Verification items for the finished model (mm, model axes). A direction names the side the tool comes from. Give positions to 0.01 mm unless a question says otherwise; leave off trailing zeros. Order: outer loops, then holes, each group sorted by start corner. A loop starts at its lowest first (then second) coordinate and runs counter-clockwise, first axis right, second up. Notation, with made-up numbers: M 43.5,-5 L 76.5,-5 A11 cw 76.5,-1 Z; hole C -32.75,26.5 d4. An arc over 180 degrees is marked long. Answer as a JSON object with one key per item and string values.
```python
from build123d import *

# Parameters (mm, degrees)
SKETCH_1_R          = 1
EXTRUDE_1_DEPTH     = 3.3
SKETCH_2_W          = 20
SKETCH_2_H          = 8
CUT_EXTRUDE_1_DEPTH = 2.2
FILLET_1_R          = 1
EXTRUDE_2_DEPTH     = 2


with BuildPart() as part:
    # 草图1 → 凸台-拉伸1 (new body)
    with BuildSketch(Plane.XY):
        with BuildLine():
            Line((10.5, -13.638181697), (10.5, -22.5))
            ThreePointArc((10.5, -22.5), (0, -33), (-10.5, -22.5))
            Line((-10.5, -22.5), (-10.5, -13.638181697))
            ThreePointArc((-10.5, -13.638181697), (-7.5, 0), (-10.5, 13.638181697))
            Line((-10.5, 13.638181697), (-10.5, 22.5))
            ThreePointArc((-10.5, 22.5), (0, 33), (10.5, 22.5))
            Line((10.5, 22.5), (10.5, 13.638181697))
            ThreePointArc((10.5, 13.638181697), (7.5, 0), (10.5, -13.638181697))
        make_face()
        with Locations((0, 7)):
            Circle(SKETCH_1_R, mode=Mode.SUBTRACT)
        with Locations((0, -7)):
            Circle(SKETCH_1_R, mode=Mode.SUBTRACT)
        with Locations((-6, 28.25)):
            Circle(SKETCH_1_R, mode=Mode.SUBTRACT)
        with Locations((6, 28.25)):
            Circle(SKETCH_1_R, mode=Mode.SUBTRACT)
        with Locations((6, -28.25)):
            Circle(SKETCH_1_R, mode=Mode.SUBTRACT)
        with Locations((-6, -28.25)):
            Circle(SKETCH_1_R, mode=Mode.SUBTRACT)
        with BuildLine():
            Line((-4, -22.499999544), (-4, -8.5))
            Line((-4, -8.5), (4, -8.5))
            Line((4, -8.5), (4, -22.500000456))
            ThreePointArc((4, -22.500000456), (-4.56e-07, -26.5), (-4, -22.499999544))
        make_face(mode=Mode.SUBTRACT)
        with BuildLine():
            Line((-4, 22.499999544), (-4, 8.5))
            Line((-4, 8.5), (4, 8.5))
            Line((4, 8.5), (4, 22.500000456))
            ThreePointArc((4, 22.500000456), (-4.56e-07, 26.5), (-4, 22.499999544))
        make_face(mode=Mode.SUBTRACT)
    extrude(amount=EXTRUDE_1_DEPTH)

    # 草图2 → 切除-拉伸1 (cut)
    with BuildSketch(Plane.XY.offset(3.3)):
        Polygon((-3.8, 24.3), (-2.871447866, 34.3), (2.871447866, 34.3), (3.8, 24.3), (8.25, 24.3), (8.25, 17.8), (-8.25, 17.8), (-8.25, 24.3), align=None)
        Rectangle(SKETCH_2_W, SKETCH_2_H)
        Polygon((3.8, -24.3), (8.25, -24.3), (8.25, -17.8), (-8.25, -17.8), (-8.25, -24.3), (-3.8, -24.3), (-2.871447866, -34.3), (2.871447866, -34.3), align=None)
    extrude(amount=-CUT_EXTRUDE_1_DEPTH, mode=Mode.SUBTRACT)

    # 圆角1
    fillet_1_edges = [part.edges().sort_by_distance(p)[0] for p in [
        (0, -4, 1.1),
        (0, 4, 1.1),
        (0, -4, 3.3),
        (0, 4, 3.3),
    ]]
    fillet(fillet_1_edges, radius=FILLET_1_R)

    # 草图3 → 凸台-拉伸2 (add)
    with BuildSketch(Plane(origin=(0, 8.5, 0), x_dir=(1, 0, 0), z_dir=(0, 1, 0))):
        with BuildLine():
            Line((-3, -3.3), (3, -3.3))
            ThreePointArc((3, -3.3), (0, -0.3), (-3, -3.3))
        make_face()
    extrude_2 = extrude(amount=EXTRUDE_2_DEPTH)

    # 镜向1: 凸台-拉伸2 across plane
    add(extrude_2.mirror(Plane.ZX))


solid = part.part
```
Q1. Section check D-D on y = -28.25. Record the cut outline in (x, z), then the cut area to 3 significant figures.
Resolved:
{"outline": "M -8.79,0 L -7,0 L -7,3.3 L -8.79,3.3 Z; M -5,0 L 5,0 L 5,3.3 L 3.43,3.3 L 3.43,1.1 L -3.43,1.1 L -3.43,3.3 L -5,3.3 Z; M 7,0 L 8.79,0 L 8.79,3.3 L 7,3.3 Z", "area": "29.7 mm²"}
Q2. Gauge pin test, flat ends, axial feed: pin 1 Ø5 at (x, y) = (2.5, -0.5) entering from +Z; pin 2 Ø1 at (y, z) = (6.5, 1) entering from +X; pin 3 Ø1.1 at (x, z) = (-6, 1.5) entering from +Y. Record the tip position at first contact, or that the pin passes through.
Resolved:
{"pin 1": "stops at z = 1.1", "pin 2": "stops at x = 8.26", "pin 3": "stops at y = 31.47"}
Q3. Material ranges on L1, parallel to Y at x = 0, z = 0.95; L2, parallel to Y at x = 6, z = 1.8; L3, parallel to X at y = 10, z = 1.35, recorded low to high.
Resolved:
{"L1": "y = -33 to -26.5, -10.5 to -8, -6 to 6, 8 to 10.5, 26.5 to 33", "L2": "y = -31.12 to -29.25, -27.25 to -24.3, -17.8 to -3.95, 3.95 to 17.8, 24.3 to 27.25, 29.25 to 31.12", "L3": "x = -9.08 to -4, -2.28 to 2.28, 4 to 9.08"}
Q4. Section check C-C on x = -2. Record the cut outline in (y, z).
Resolved:
{"outline": "M -32.81,0 L -25.96,0 L -25.96,1.1 L -32.81,1.1 Z; M -10.5,1.06 L -8.5,1.06 L -8.5,0 L 8.5,0 L 8.5,1.06 L 10.5,1.06 L 10.5,3.3 L 5,3.3 A1 ccw 4,2.3 L 4,2.1 A1 cw 3,1.1 L -3,1.1 A1 cw -4,2.1 L -4,2.3 A1 ccw -5,3.3 L -10.5,3.3 Z; M 25.96,0 L 32.81,0 L 32.81,1.1 L 25.96,1.1 Z"}
Q5. Section check A-A on x = -9. Record the cut outline in (y, z).
Resolved:
{"outline": "M -27.91,0 L -9.76,0 L -9.76,3.3 L -27.91,3.3 Z; M 9.76,0 L 27.91,0 L 27.91,3.3 L 9.76,3.3 Z"}
Q6. Section check B-B on y = -11.5. Record the cut outline in (x, z), then the cut area to 3 significant figures.
Resolved:
{"outline": "M -9.6,0 L -4,0 L -4,3.3 L -9.6,3.3 Z; M 4,0 L 9.6,0 L 9.6,3.3 L 4,3.3 Z", "area": "37.0 mm²"}
Q7. Release check for a two-part mould opening along Y. For faces 1 (the face through (0.2, -33, 0.9)), 2 (the face through (-4, -14, 2)) record: +Y half, -Y half, draft (parallel to the pull), parting line (faces both ways), or undercut.
Resolved:
{"face 1": "-Y half", "face 2": "undercut"}
Q8. Tool access check on faces 3 (the face through (0, 10.5, 2)), 4 (the face through (6, -17.8, 2)), 5 (the face through (0.1, -9.5, 0.3)). Record the directions out of +Z, -Z, +X, -X, +Y, -Y that give a thin tool (end or side, any length) a straight path to the whole face; none if there is none.
Resolved:
{"face 3": "+Z, -Z", "face 4": "+Z", "face 5": "-Z"}
